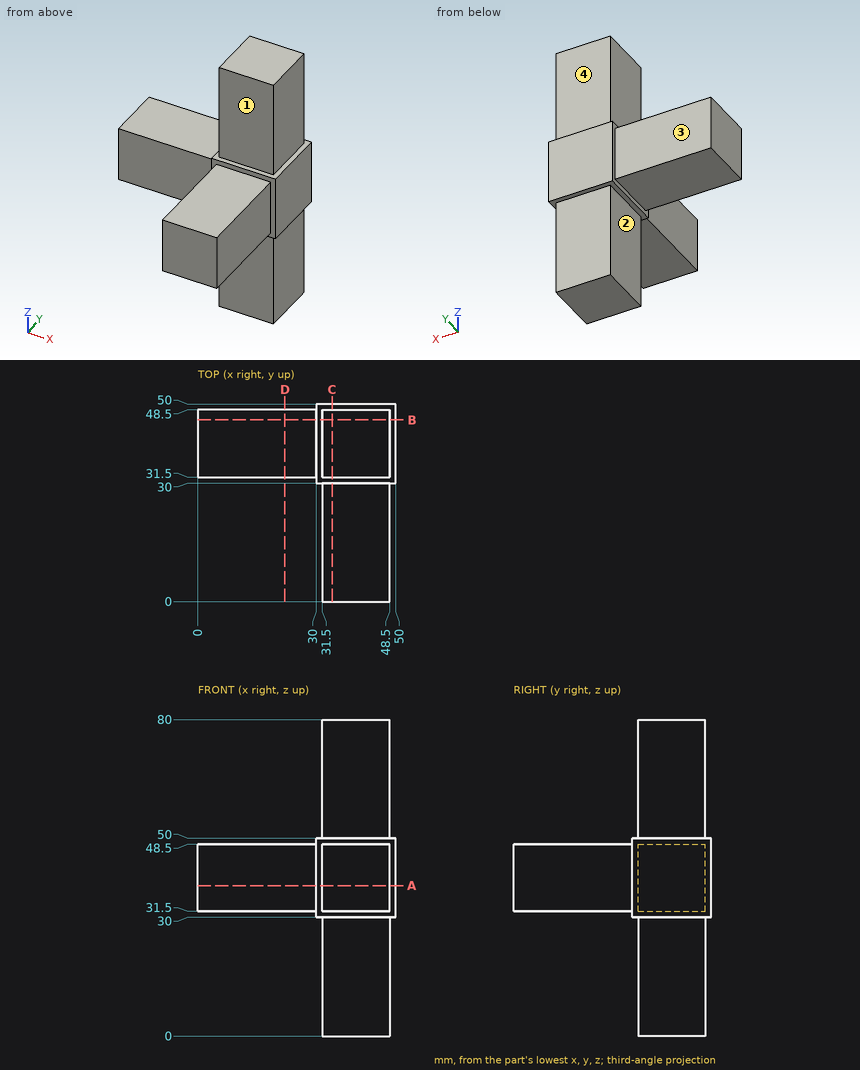
Input: dimensioned drawing with shaded views. Units: mm. Origin: part minimum x, y, z. A direction names the side the tool comes from. Round coordinates to 2 decimals unless told otherwise and drop trailing zeros. Order: outer loops, then holes, each group sorted by start corner. A loop starts at its lowest first (then second) coordinate and runs counter-clockwise, first axis right, second up. Notation, with made-up numbers: M 49.25,-31.5 L 106.25,-31.5 A24 cw 106.25,1.5 Z; hole C -0.5,-33.5 d10. An arc over 180 degrees is marked long. Use one line per item in the form item = value. Start each with the question number.
Q1. Cut plane B-B (y = 46). Return loops of the section in (x, z).
Q2. Cut plane A-A (z = 38). Return loops of the section in (x, y), and give its area (3 significant figures).
Q3. Material intervals for line 1 (Y direction, x = 34.5, z = 14), sorted ascending. Write a range as [from, to].
Q4. Access query for the marked faces 1, 2, 3 and 4. Directions: +Z, -Z, +X, -X, +Y, -Y. A direction counts if a zero-diameter tool reaches every point of the face in a straight line with its end or side. Return the directions, or none.
Q5. Pin query (flat end, axial travel): pin 1 Ø5 at (x, y) = (41.5, 8.5) entering from +Z; pin 2 Ø18.5 at (x, z) = (12, 41.5) entering from +Y; pin 3 Ø5 at (x, y) = (16.5, 36.5) entering from -Z; pin 4 Ø12 at (x, y) = (44.5, 38.5) entering from -Z. Return the tip coordinate at first contact, or that it passes through.
Q6. Cut plane D-D (x = 22). Return loops of the section in (y, z).
Geometry results:
q1.outline = M 0,31.5 L 30,31.5 L 30,30 L 31.5,30 L 31.5,0 L 48.5,0 L 48.5,30 L 50,30 L 50,50 L 48.5,50 L 48.5,80 L 31.5,80 L 31.5,50 L 30,50 L 30,48.5 L 0,48.5 Z
q2.outline = M 0,31.5 L 30,31.5 L 30,30 L 31.5,30 L 31.5,0 L 48.5,0 L 48.5,30 L 50,30 L 50,50 L 30,50 L 30,48.5 L 0,48.5 Z
q2.area = 1,420 mm^2
q3.line_1 = [31.5, 48.5]
q4.face_1 = +Z, +X, -X, -Y
q4.face_2 = -Z, -X, +Y, -Y
q4.face_3 = +Z, -Z, -X, +Y
q4.face_4 = +Z, +X, -X, +Y
q5.pin_1 = 48.5
q5.pin_2 = 48.5
q5.pin_3 = 31.5
q5.pin_4 = 0
q6.outline = M 31.5,31.5 L 48.5,31.5 L 48.5,48.5 L 31.5,48.5 Z
